Geometry: final body of the model. Coordinates: model frame, mm. Face numbers are marked on the shaded views. A direction names the side the tool comes from. Give positions to 0.01 mm unless a question says otherwise; leave off trailing zeros. Order: outer loops, then holes, each group sorted by start corner. A loop starts at its lowest first (then second) coordinate and runs counter-clockwise, first axis right, second up. Notation, with made-up numbers: (14, -16) - (36, -16) arc R23 ccw to (36, 9) - close; hole circle Ø2 at (12.5, 41). An arc over 180 degrees is marked (long way). Use one line per item in the form item = value.
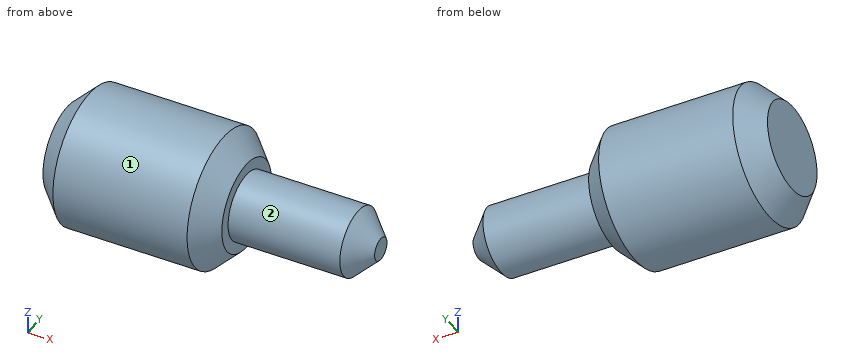
Autodesk Inventor part; units mm, degrees
ref_plane "YZ Plane" through (0, 0, 0) normal (1, 0, 0) x (0, 1, 0)
ref_plane "XZ Plane" through (0, 0, 0) normal (0, 1, 0) x (-1, 0, 0)
ref_plane "XY Plane" through (0, 0, 0) normal (0, 0, 1) x (1, 0, 0)
sketch "Skizze1" plane through (0, 0, 0) normal (0, 0, 1) x (1, 0, 0)
  line L0 (-16.8, 0) -> (2.8, 0)
  line L1 (0, -0.6) -> (0, 3.6)
  line L2 (0, 1.5) -> (-6, 1.5)
  line L3 (-6, 1.5) -> (-6, 3)
  line L4 (-6, 3) -> (-14, 3)
  line L5 (-14, 3) -> (-14, 0)
  line L6 (-14, 0) -> (0, 0)
  line L7 (0, 0) -> (0, 1.5)
  dimension "d0" = 3
  dimension "d1" = 6
  dimension "d2" = 6
  dimension "d3" = 8
revolve "Umdrehung1" add sketch "Skizze1" angle 360 about axis through (-10, 0, 0) along (1, 0, 0)
thread "Gewinde1"
thread "Gewinde2"
chamfer "Fase1" distance 1 angle 45 3 edges at (-14, -3, 0) (-6, -3, 0) (0, -1.5, 0)
properties part number "13_1087_017"
(1) Contact query for a flat-ended pin moving along its axis: pin 1 Ø1 at (x, y) = (-8, -1) entering from -Z. Output: stop coordinate, or through.
Computed values:
pin_1 = -2.96
(2) Ray query, line 1 along X through (y, z) = (0.05, -1.9); line 2 along Z through (x, y) = (-10.5, 0.1); line 3 along Y through (x, z) = (-13.5, 2.15). Return the intervals inside material, ascending.
Computed values:
line_1 = -14 to -6
line_2 = -3 to 3
line_3 = -1.28 to 1.28
(3) Cut plane C-C on x = -8.5. Output: boundary loops of the cut face in (y, z), plus the area to 3 significant figures.
Computed values:
outline = circle Ø6 at (0, 0)
area = 28.3 mm²
(4) Cut plane A-A on z = 0. Output: boundary loops of the cut face in (x, y).
Computed values:
outline = (-14, -2) - (-13, -3) - (-7, -3) - (-6, -2) - (-6, -1.5) - (-1, -1.5) - (0, -0.5) - (0, 0.5) - (-1, 1.5) - (-6, 1.5) - (-6, 2) - (-7, 3) - (-13, 3) - (-14, 2) - close
(5) Reachability of the marked faces 1 and 2 from +Z, -Z, +X, -X, +Y, -Y: full face, straight path, thin tool, end or side. Return the list, or none.
Computed values:
face_1 = +X, -X
face_2 = +X
